```python
from build123d import *
from build123d.topology import SkipClean

# Parameters (mm, degrees)
SKETCH1_R           = 2
BOSS_EXTRUDE1_DEPTH = 5.5
SKETCH2_R           = 6.5
SKETCH2_R_2         = 2
BOSS_EXTRUDE3_DEPTH = 5


with BuildPart() as part:
    # Sketch1 → Boss-Extrude1 (new body)
    with BuildSketch(Plane(origin=(0, 0, 0), x_dir=(0, 0, -1), z_dir=(1, 0, 0))):
        with BuildLine():
            Line((4.437059837, 4.75), (145.562940163, 4.75))
            ThreePointArc((145.562940163, 4.75), (156.5, 0), (145.562940163, -4.75))
            Line((145.562940163, -4.75), (4.437059837, -4.75))
            ThreePointArc((4.437059837, -4.75), (-6.5, 0), (4.437059837, 4.75))
        make_face()
        Circle(SKETCH1_R, mode=Mode.SUBTRACT)
        with Locations((150, 0)):
            Circle(SKETCH1_R, mode=Mode.SUBTRACT)
    extrude(amount=BOSS_EXTRUDE1_DEPTH)

    # Sketch2 → Boss-Extrude3 (add)
    with SkipClean():  # the faces are left unmerged after this step: merging them gives an invalid solid
        with BuildSketch(Plane(origin=(5.5, 0, 0), x_dir=(0, 0, -1), z_dir=(1, 0, 0))):
            with Locations(Location((150, 0, 0), (0, 0, 226.9509202))):
                Circle(SKETCH2_R)
            with Locations((150, 0)):
                Circle(SKETCH2_R_2, mode=Mode.SUBTRACT)
        extrude(amount=BOSS_EXTRUDE3_DEPTH)


solid = part.part
```
Input: part model. Units: mm. Frame: model coordinates. A direction names the side the tool comes from. Give positions to 0.01 mm unless a question says otherwise; leave off trailing zeros. Order: outer loops, then holes, each group sorted by start corner. A loop starts at its lowest first (then second) coordinate and runs counter-clockwise, first axis right, second up. Notation, with made-up numbers: M 37,-2 L 77,-2 A24 cw 77,23 Z; hole C 60,-13 d4. An arc over 180 degrees is marked long. Return JSON: item names as keys, results as strings.
1) Line query: L1, parallel to Y at x = 3.3, z = 0; L2, parallel to X at y = 2.5, z = -64; L3, parallel to Y at x = 1.5, z = -136.5. Output: solid intervals per line, ascending. Write a range as [from, to].
Taken from the geometry:
{"L1": "y = [-6.5, -2], [2, 6.5]", "L2": "x = [0, 5.5]", "L3": "y = [-4.75, 4.75]"}
2) Contact query for flat-ended pins moving along their axis: pin 1 (5 mm diameter, centred on x = 6.5, z = -79, fed in from +Y); pin 2 (3 mm diameter, centred on y = 0, z = 0, fed in from -X); pin 3 (3 mm diameter, centred on x = 2.5, z = -66.5, fed in from -Y); pin 4 (1.5 mm diameter, centred on x = 6, y = -2.5, fed in from -Z). Output: stop coordinate, or through.
Taken from the geometry:
{"pin 1": "stops at y = 4.75", "pin 2": "passes through", "pin 3": "stops at y = -4.75", "pin 4": "stops at z = -156.26"}
3) Section query A-A on z = -150. Output: boundary loops of the cut face in (x, y).
Taken from the geometry:
{"outline": "M 0,-6.5 L 10.5,-6.5 L 10.5,-2 L 0,-2 Z; M 0,2 L 10.5,2 L 10.5,6.5 L 0,6.5 Z"}
4) Section query B-B on x = 8.75. Output: boundary loops of the cut face in (y, z), and give its area (3 significant figures).
Taken from the geometry:
{"outline": "C 0,-150 d13; hole C 0,-150 d4", "area": "120 mm2"}
5) Mould query, pull axis Z, two halves, no side actions, for faces 3 (the face through (5.5, 0, -71)), 4 (the face through (3, -4.75, -76)), 5 (the face through (5, 0, -148)). Classes: released by +Z, released by -Z, zero draft, split by the parting line, or undercut.
Taken from the geometry:
{"face 3": "zero draft", "face 4": "undercut", "face 5": "undercut"}
6) Section query D-D on z = -87. Output: boundary loops of the cut face in (x, y), and give its area (4 significant figures).
Taken from the geometry:
{"outline": "M 0,-4.75 L 5.5,-4.75 L 5.5,4.75 L 0,4.75 Z", "area": "52.25 mm2"}
7) Access query for faces 1 (the face through (2.712, -0.211, 6.497)), 2 (the face through (3, 4.75, -74)). Directions: +Z, -Z, +X, -X, +Y, -Y. A direction counts if a zero-diameter tool reaches every point of the face in a straight line with its end or side. Return the directions, or none.
Taken from the geometry:
{"face 1": "+X, -X", "face 2": "+X, -X, +Y"}
8) Section query C-C on z = 0. Output: boundary loops of the cut face in (x, y), and give its area (3 significant figures).
Taken from the geometry:
{"outline": "M 0,-6.5 L 5.5,-6.5 L 5.5,-2 L 0,-2 Z; M 0,2 L 5.5,2 L 5.5,6.5 L 0,6.5 Z", "area": "49.5 mm2"}
